Input: part model. Units: mm. Frame: model coordinates. Coordinates: 2 decimals unless noted, no trailing zeros. Order: outer loops, then holes, each group sorted by start corner. A loop starts at its lowest first (then second) coordinate and runs counter-clockwise, first axis right, second up. Notation, with made-up numbers: (7, 37.25) -> (57, 37.25) arc R32 cw to (57, 63.25) -> close; hole circle Ø9 at (-25, -37). An arc over 180 degrees is marked (long way). Answer as CSV lines item,"result".
Autodesk Inventor part; units mm, degrees
ref_plane "YZ Plane" through (0, 0, 0) normal (1, 0, 0) x (0, 1, 0)
ref_plane "XZ Plane" through (0, 0, 0) normal (0, 1, 0) x (-1, 0, 0)
ref_plane "XY Plane" through (0, 0, 0) normal (0, 0, 1) x (1, 0, 0)
sketch "スケッチ1" plane through (0, 0, 0) normal (0, 0, 1) x (1, 0, 0)
  line L0 (-2.5294, 6.0706) -> (-2.5294, -17.9294)
  line L1 (-2.5294, -17.9294) -> (-7.5294, -17.9294)
  line L2 (-7.5294, -17.9294) -> (-7.5294, 6.0706)
  arc A0 (-6.2794, 6.0706) -> (-3.2794, 6.0706) centre (-4.7794, 6.0706) ccw
  line L3 (-7.5294, 6.0706) -> (-6.2794, 6.0706)
  line L4 (-3.2794, 6.0706) -> (-2.5294, 6.0706)
  point P0 (0, 0)
  dimension "d0" = 5
  dimension "d3" = 3
revolve "回転1" add sketch "スケッチ1" angle 360 about axis through (-2.5294, -17.9294, 0) along (-1, 0, 0)
sketch "スケッチ2" plane through (-2.5294, -17.9294, 0) normal (1, 0, 0) x (0, 0, -1)
  circle A0 centre (0, 0) radius 24
  circle A1 centre (0, 0) radius 14
  circle A2 centre (-14, 0) radius 1.5
  circle A3 centre (14, 0) radius 1.5
  circle A4 centre (0, -14) radius 1.5
  circle A5 centre (0, 14) radius 1.5
  point P0 (0, 17.9294)
  dimension "d5" = 28
  dimension "d7" = 3
  dimension "d8" = 3
  dimension "d9" = 3
  dimension "d10" = 3
hole "穴1" at (-2.5294, -3.9294, 0) at (-2.5294, -17.9294, 14) at (-2.5294, -31.9294, 0) at (-2.5294, -17.9294, -14) direction (-1, 0, 0) diameter 2.459 end through all
sketch "スケッチ3" plane through (-2.5294, -17.9294, 0) normal (1, 0, 0) x (0, 0, -1)
  circle A0 centre (0, 0) radius 24
  circle A1 centre (0, 0) radius 2.5
  point P0 (0, 17.9294)
  dimension "d18" = 5
hole "穴2" at (-2.5294, -17.9294, 0) direction (-1, 0, 0) diameter 5 end through all
properties part number "hoiiru" material "アルミニウム 6061-O"
1. Mould query, pull axis Y, two halves, no side actions, for faces 1 (the face through (-2.899, -36.975, -14.604)), 2 (the face through (-5.064, -20.408, 0.325)), 3 (the face through (-7.529, -18, 5)). Classes: released by +Y, released by -Y, zero draft, split by the parting line, or undercut.
Findings:
face 1,"split by the parting line"
face 2,"undercut"
face 3,"zero draft"
2. Cut plane B-B (x = -4.3). Return the cut outline in (y, z), plus the area to 3 significant figures.
Findings:
outline,"circle Ø45.16 at (-17.93, 0); hole circle Ø2.46 at (-31.93, 0); hole circle Ø5 at (-17.93, 0); hole circle Ø2.46 at (-17.93, -14); hole circle Ø2.46 at (-17.93, 14); hole circle Ø2.46 at (-3.93, 0)"
area,"1,560 mm2"
3. Ray query, line 1 along Y through (x, z) = (-4.2, 0); line 2 along Y through (x, z) = (-5.4, 0) (3 decimals); line 3 along Z through (x, y) = (-6.1, -18). Return the intervals inside material, ascending.
Findings:
line 1,"y = -40.55 to -33.16, -30.7 to -20.43, -15.43 to -5.16, -2.7 to 4.69"
line 2,"y = -40.564 to -33.159, -30.7 to -20.429, -15.429 to -5.159, -2.7 to 4.705"
line 3,"z = -23.29 to -15.23, -12.77 to -2.5, 2.5 to 12.77, 15.23 to 23.29"
4. Contact query for flat-ended pins moving along their axis: pin 1 (1.5 mm diameter, centred on x = -6.5, z = 15.5, fed in from -Y); pin 2 (1.5 mm diameter, centred on x = -7, z = 4.5, fed in from -Y); pin 3 (3 mm diameter, centred on x = -4.5, y = -27, fed in from +Z); pin 4 (2 mm diameter, centred on y = -17.93, z = 14, fed in from +X). Output: stop coordinate, or through.
Findings:
pin 1,"stops at y = -36.86"
pin 2,"stops at y = -41.63"
pin 3,"stops at z = 22.56"
pin 4,"passes through"
5. Cut plane A-A (z = 0). Return the cut outline in (x, y).
Findings:
outline,"(-7.53, -41.93) -> (-6.28, -41.93) arc R1.5 cw to (-3.28, -41.93) -> (-2.53, -41.93) -> (-2.53, -33.16) -> (-7.53, -33.16) -> close; (-7.53, -30.7) -> (-2.53, -30.7) -> (-2.53, -20.43) -> (-7.53, -20.43) -> close; (-7.53, -15.43) -> (-2.53, -15.43) -> (-2.53, -5.16) -> (-7.53, -5.16) -> close; (-7.53, -2.7) -> (-2.53, -2.7) -> (-2.53, 6.07) -> (-3.28, 6.07) arc R1.5 cw to (-6.28, 6.07) -> (-7.53, 6.07) -> close"
